Geometry check sheet. Reference: the model listing, model coordinates, mm. Face numbers are marked on the shaded views. A direction names the side the tool comes from. Coordinates: 2 decimals unless noted, no trailing zeros. Write each loop counter-clockwise with the first axis right and the second up, starting at its lowest first coordinate (ties: lowest second). Pieces come first, ordered by that corner, then holes. Notation, with made-up numbers: (-36, 84) -> (-29, 84) arc R18 ccw to (-29, 115) -> close; hole circle Ø5 at (70, -26.75). An arc over 180 degrees is marked (long way). Put each result on its own line as item: value. Start each with the question number.
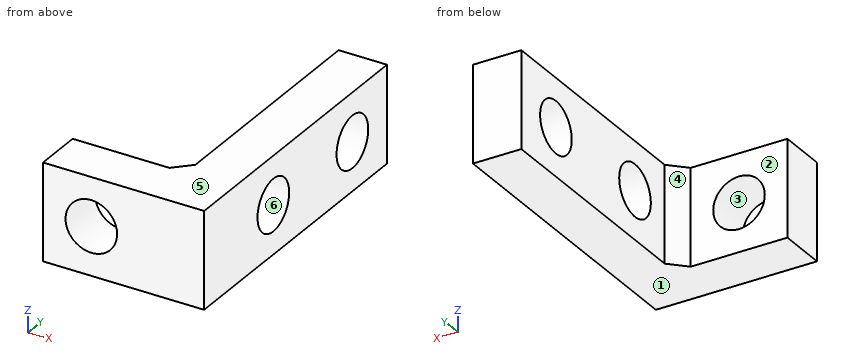
from build123d import *

# Parameters (mm, degrees)
SKETCH1_W           = 10
SKETCH1_H           = 6
SKETCH1_R           = 1.6
BOSS_EXTRUDE1_DEPTH = 3
SKETCH2_W           = 3
SKETCH2_H           = 6
BOSS_EXTRUDE2_DEPTH = 15.5
SKETCH3_R           = 1.6
CUT_EXTRUDE1_DEPTH  = 21.006249024
BOSS_EXTRUDE3_DEPTH = 6


with BuildPart() as part:
    # Sketch1 → Boss-Extrude1 (new body)
    with BuildSketch(Plane(origin=(0, 0, 0), x_dir=(1, 0, 0), z_dir=(0, 1, 0))):
        Rectangle(SKETCH1_W, SKETCH1_H)
        with Locations(Location((-2, 0, 0), (0, 0, 270))):
            Circle(SKETCH1_R, mode=Mode.SUBTRACT)
    extrude(amount=BOSS_EXTRUDE1_DEPTH)

    # Sketch2 → Boss-Extrude2 (add)
    with BuildSketch(Plane(origin=(0, 3, 0), x_dir=(1, 0, 0), z_dir=(0, 1, 0))):
        with Locations((3.5, 0)):
            Rectangle(SKETCH2_W, SKETCH2_H)
    extrude(amount=BOSS_EXTRUDE2_DEPTH)

    # Sketch3 → Cut-Extrude1 (cut, through all)
    with BuildSketch(Plane.ZY.offset(-2)):
        with Locations((0, 7)):
            Circle(SKETCH3_R)
        with Locations((0, 15)):
            Circle(SKETCH3_R)
    extrude(amount=-CUT_EXTRUDE1_DEPTH, mode=Mode.SUBTRACT)

    # Sketch5 → Boss-Extrude3 (add)
    with BuildSketch(Plane(origin=(2, 3, 3), x_dir=(1, 0, 0), z_dir=(0, 0, 1))):
        Polygon((-1, 0), (0, 1), (0, 0), align=None)
    extrude(amount=-BOSS_EXTRUDE3_DEPTH)


solid = part.part
Item 1: Go/stop test with flat-tipped pins: P1, Ø3, axis at x = -2, z = 0, coming from the -Y side; P2, Ø1.8, axis at x = -1.5, z = -1.5, coming from the +Y side; P3, Ø1.5, axis at x = 1, z = -2.5, coming from the +Y side. Record where each tip stops, or that it passes through.
Item 2: Section check B-B, the plane y = 7. Enter the section's corners in (x, z).
Item 3: Scan lines: line 1 along Y through (x, z) = (3.6, 0); line 2 along X through (y, z) = (0.7, 0); line 3 along Y through (x, z) = (-0.75, -2.65). Record each from-to range of solid material in increasing order. Write a range as [from, to].
Item 4: Section check A-A, the plane x = -2. Enter the section's corners in (y, z).
Item 5: Mould release check, pull along Z, two halves, no side actions. Record for the marked faces 3, 4, 5 and 6: released by +Z, released by -Z, zero draft, split by the parting line, or undercut.
Item 6: Section check D-D, the plane z = 2.55. Enter the section's corners in (x, y), and give its area (3 significant figures).
Item 7: Access from +Z, -Z, +X, -X, +Y, -Y to the whole of each face (thin tool, end or side, straight path). Record for the marked faces 1 and 2.
Item 8: Section check C-C, the plane z = 0.6. Enter the section's corners in (x, y).
From the geometry:
1. P1: through
1. P2: y = 3
1. P3: y = 3.75
2. outline: (2, -3) -> (5, -3) -> (5, -1.6) -> (2, -1.6) -> close; (2, 1.6) -> (5, 1.6) -> (5, 3) -> (2, 3) -> close
3. line 1: [0, 5.4], [8.6, 13.4], [16.6, 18.5]
3. line 2: [-5, -3.6], [-0.4, 5]
3. line 3: [0, 3]
4. outline: (0, -3) -> (3, -3) -> (3, -1.6) -> (0, -1.6) -> close; (0, 1.6) -> (3, 1.6) -> (3, 3) -> (0, 3) -> close
5. face 3: undercut
5. face 4: zero draft
5. face 5: released by +Z
5. face 6: undercut
6. outline: (-5, 0) -> (5, 0) -> (5, 18.5) -> (2, 18.5) -> (2, 4) -> (1, 3) -> (-5, 3) -> close
6. area: 77.0 mm²
7. face 1: -Z, +X, -X, +Y, -Y
7. face 2: +Z, -Z, -X, +Y
8. outline: (-5, 0) -> (-3.48, 0) -> (-3.48, 3) -> (-5, 3) -> close; (-0.52, 0) -> (5, 0) -> (5, 5.52) -> (2, 5.52) -> (2, 4) -> (1, 3) -> (-0.52, 3) -> close; (2, 8.48) -> (5, 8.48) -> (5, 13.52) -> (2, 13.52) -> close; (2, 16.48) -> (5, 16.48) -> (5, 18.5) -> (2, 18.5) -> close
